The listing builds one solid part. Answer for the finished solid, in the listing's coordinates (mm). A direction names the side the tool comes from. Coordinates: 2 decimals unless noted, no trailing zeros. Loops run counter-clockwise (first coordinate to the right, second up) from the corner with the lowest first, then second, coordinate; pieces in that order, holes last. Notation, with made-up numbers: M 74.5,47.25 L 107.5,47.25 A19 ccw 107.5,64.25 Z; hole C 16,61 d4. An arc over 180 degrees is marked long. Answer as CSV lines item,"result". Start each with the question number.
```python
from build123d import *

# Parameters (mm, degrees)
SKETCH2_R           = 1.75
SKETCH2_R_2         = 2.5
BOSS_EXTRUDE1_DEPTH = 15
SPLIT1_START        = -15
SPLIT1_DEPTH        = 30


# Read off the part's stored shape, not the designer's step: Split1
with BuildPart() as part:
    # Sketch2 → Boss-Extrude1 (new, symmetric)
    with BuildSketch(Plane.XY):
        with BuildLine():
            Line((0, 10), (50, 10))
            Line((50, 10), (110, -50))
            ThreePointArc((110, -50), (109.927822148, -62.57300177), (97.356477729, -62.356477729))
            Line((97.356477729, -62.356477729), (45, -10))
            Line((45, -10), (0, -10))
            ThreePointArc((0, -10), (-10, 0), (0, 10))
        make_face()
        Circle(SKETCH2_R, mode=Mode.SUBTRACT)
        with Locations((103.749176054, -56.250823946)):
            Circle(SKETCH2_R_2, mode=Mode.SUBTRACT)
    extrude(amount=BOSS_EXTRUDE1_DEPTH, both=True)

    # Split1 outline → Split1 (cut)
    with BuildSketch(Plane.XY.offset(SPLIT1_START)):
        with BuildLine():
            ThreePointArc((111.20911577, -51.507945133), (108.320634217, -60.472229721), (99.61434242, -64.06419395))
            ThreePointArc((99.61434242, -64.06419395), (110.24370673, -62.248045911), (111.20911577, -51.507945133))
        make_face()
    extrude(amount=SPLIT1_DEPTH, mode=Mode.SUBTRACT)


solid = part.part
```
Item 1: Section D-D on y = -42 is taken. Determine the outline of the cut face in (x, z), then the cut area to 3 significant figures.
Item 2: Consider line 1 (Y direction, x = 0, z = 4.75); line 2 (Y direction, x = 39, z = -1.5); line 3 (X direction, y = 1, z = 9.5). Determine where each line is inside the solid, lowest interval first.
Item 3: For a pull along X with two mould halves and no side action, classify faces 3 (the face through (1.617, -0.67, -0.21)), 4 (the face through (25, 10, 0)), 5 (the face through (72, -37, 0)) as pulls with the +X half, pulls with the -X half, needs draft (parallel to the pull), parting line crosses it, or undercut.
Item 4: Each of these flat-tipped pins is pushed along its axis until it touches: P1, Ø10, axis at x = 43.5, z = -9, coming from the -Y side; P2, Ø6, axis at y = -17, z = 6, coming from the -X side; P3, Ø10, axis at y = -14.5, z = 6, coming from the +X side. Where does it stop, or does it pass through?
Item 5: Section B-B on z = 3 is taken. Determine the outline of the cut face in (x, y), then the cut area to 3 significant figures.
Item 6: Section A-A on y = 0 is taken. Determine the outline of the cut face in (x, z), then the cut area to 4 significant figures.
Item 7: Section C-C on x = 75 is taken. Determine the outline of the cut face in (y, z).
Item 8: For faces 1 (the face through (55, -16, 15)), 2 (the face through (23, -10, 0)), determine the directions among +Z, -Z, +X, -X, +Y, -Y from which every point of the face is accessible in a straight line to the end or side of a thin tool.
Results are:
1,outline,"M 77,-15 L 102,-15 L 102,15 L 77,15 Z"
1,area,"750 mm²"
2,line 1,"-10 to -1.75, 1.75 to 10"
2,line 2,"-10 to 10"
2,line 3,"-9.95 to -1.44, 1.44 to 59"
3,face 3,"undercut"
3,face 4,"needs draft"
3,face 5,"pulls with the -X half"
4,P1,"y = -13.5"
4,P2,"x = 49"
4,P3,"x = 79.5"
5,outline,"M 0,-10 L 45,-10 L 97.36,-62.36 A8.84 ccw 99.61,-64.06 A11.2 ccw 111.21,-51.51 A8.84 ccw 110,-50 L 50,10 L 0,10 A10 ccw Z; hole C 0,0 d3.5; hole C 103.75,-56.25 d5"
5,area,"2,570 mm²"
6,outline,"M -10,-15 L -1.75,-15 L -1.75,15 L -10,15 Z; M 1.75,-15 L 60,-15 L 60,15 L 1.75,15 Z"
6,area,"1,995 mm²"
7,outline,"M -40,-15 L -15,-15 L -15,15 L -40,15 Z"
8,face 1,"+Z, +X, -X, +Y, -Y"
8,face 2,"+Z, -Z, -X, -Y"
